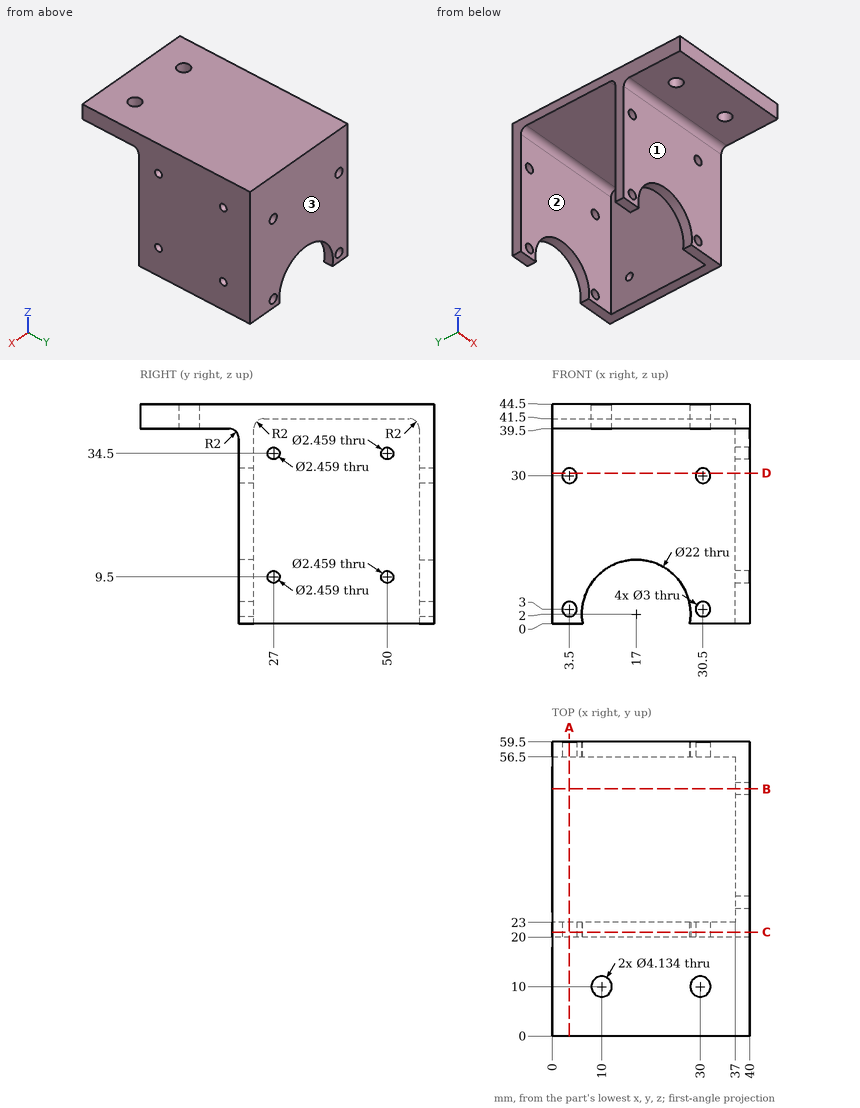
Check sheet for the drawn part. Datum: minimum x, y, z corner. Units: mm. A direction names the side the tool comes from. Coordinates: 2 decimals unless noted, no trailing zeros. Loops run counter-clockwise (first coordinate to the right, second up) from the corner with the lowest first, then second, coordinate; pieces in that order, holes last. Notation, with made-up numbers: M -28,28 L 16,28 A19 ccw 16,54 Z; hole C 71,9 d10. An arc over 180 degrees is marked long. Answer as a JSON object with one key per item and string values.
1. Sectioned sample at D-D on z = 30.5. Record the cut outline in (x, y).
Outcome:
{"outline": "M 0,20 L 2.09,20 L 2.09,23 L 0,23 Z; M 0,56.5 L 2.09,56.5 L 2.09,59.5 L 0,59.5 Z; M 4.91,20 L 29.09,20 L 29.09,23 L 4.91,23 Z; M 4.91,56.5 L 29.09,56.5 L 29.09,59.5 L 4.91,59.5 Z; M 31.91,20 L 40,20 L 40,59.5 L 31.91,59.5 L 31.91,56.5 L 37,56.5 L 37,23 L 31.91,23 Z"}
2. Sectioned sample at A-A on x = 3.5. Count the separate pieces of the cut face and the enclosed holes in it, and give its area (3 significant figures).
Outcome:
{"separate pieces": "5", "enclosed holes": "0", "area": "434 mm²"}
3. Sectioned sample at C-C on y = 21. Record the cut outline in (x, z).
Outcome:
{"outline": "M 0,0 L 6.18,0 A11 cw long 27.82,0 L 40,0 L 40,44.5 L 0,44.5 Z; hole C 3.5,3 d3; hole C 3.5,30 d3; hole C 30.5,3 d3; hole C 30.5,30 d3"}
4. Depth check by flat-ended pin: P1, Ø3, axis at y = 38, z = 6, coming from the -X side; P2, Ø3, axis at y = 27, z = 34.5, coming from the +X side; P3, Ø2.5, axis at x = 3.5, z = 3, coming from the -Y side; P4, Ø12, axis at x = 26, z = 30, coming from the -Y side. Enter the tip coordinate at first touch or a pass-through.
Outcome:
{"P1": "x = 37", "P2": "x = 40", "P3": "through", "P4": "y = 20"}
5. Scan lines: L1, parallel to Y at x = 38, z = 34.5; L2, parallel to Y at x = 8.5, z = 29; L3, parallel to Z at x = 3, y = 58. Record each from-to range of solid material in increasing order. Write a range as from..to.
Outcome:
{"L1": "20..25.77, 28.23..48.77, 51.23..59.5", "L2": "20..23, 56.5..59.5", "L3": "0..1.59, 4.41..28.59, 31.41..44.5"}
6. Access from +Z, -Z, +X, -X, +Y, -Y to the whole of each face (thin tool, end or side, straight path). Record for the marked faces 1, 2 and 3.
Outcome:
{"face 1": "-Z, +X, -X, -Y", "face 2": "-Z, -X", "face 3": "+Z, -Z, +X, -X, +Y"}
7. Sectioned sample at B-B on y = 50. Record the cut outline in (x, z), and give its area (3 significant figures).
Outcome:
{"outline": "M 0,41.5 L 37,41.5 L 37,35.73 L 40,35.73 L 40,44.5 L 0,44.5 Z; M 37,0 L 40,0 L 40,8.27 L 37,8.27 Z; M 37,10.73 L 40,10.73 L 40,33.27 L 37,33.27 Z", "area": "230 mm²"}
